Autodesk Inventor part; units mm, degrees
ref_plane "YZ Plane" through (0, 0, 0) normal (1, 0, 0) x (0, 1, 0)
ref_plane "XZ Plane" through (0, 0, 0) normal (0, 1, 0) x (-1, 0, 0)
ref_plane "XY Plane" through (0, 0, 0) normal (0, 0, 1) x (1, 0, 0)
sketch "Sketch1" plane through (0, 0, 0) normal (0, 0, 1) x (1, 0, 0)
  line L0 (0, 0) -> (70, 0)
  line L1 (70, 0) -> (70, 134)
  line L2 (70, 134) -> (0, 134)
  line L3 (0, 134) -> (0, 0)
  dimension "d0" = 70
  dimension "d1" = 134
extrude "Extrusion1" add sketch "Sketch1" along normal blind 3
sketch "Sketch2" plane through (0, 0, 3) normal (0, 0, 1) x (1, 0, 0)
  line L0 (70, 134) -> (0, 134)
  line L1 (0, 134) -> (24, 134)
  line L2 (24, 134) -> (24, 119)
  line L3 (24, 119) -> (0, 119)
  line L4 (0, 119) -> (0, 134)
  line L5 (0, 0) -> (24, 0)
  line L6 (24, 0) -> (24, 15)
  line L7 (24, 15) -> (0, 15)
  line L8 (0, 15) -> (0, 0)
  dimension "d4" = 24
  dimension "d5" = 15
  dimension "d6" = 24
  dimension "d7" = 15
extrude "Extrusion2" add sketch "Sketch2" along normal blind 37
sketch "Sketch3" plane through (0, 0, 40) normal (0, 0, 1) x (1, 0, 0)
  line L0 (24, 134) -> (0, 134) construction
  line L1 (0, 134) -> (0, 119) construction
  line L2 (0, 119) -> (24, 119) construction
  line L3 (24, 119) -> (24, 134) construction
  line L4 (0, 0) -> (24, 0) construction
  line L5 (24, 0) -> (24, 15) construction
  line L6 (24, 15) -> (0, 15) construction
  line L7 (0, 15) -> (0, 0) construction
  circle A0 centre (12, 126.5) radius 1.5
  circle A1 centre (12, 7.5) radius 1.5
  point P0 (24, 126.5)
  point P1 (24, 7.5)
  point P2 (12, 15)
  point P3 (12, 119)
  dimension "d10" = 3
  dimension "d11" = 3
extrude "Extrusion3" cut sketch "Sketch3" against normal through all
sketch "Sketch4" plane through (0, 0, 0) normal (0, 0, -1) x (-1, 0, 0)
  circle A0 centre (-12, 126.5) radius 1.5
  circle A1 centre (-12, 7.5) radius 1.5
  circle A2 centre (-12, 126.5) radius 4
  circle A3 centre (-12, 7.5) radius 4
  point P0 (0, 0)
  dimension "d14" = 8
  dimension "d15" = 8
extrude "Extrusion4" cut sketch "Sketch4" against normal blind 35 contours A0 | A1 | A2 | A3
properties part number "BP009" material "ABS Plastic"
Input: part model. Units: mm. Frame: model coordinates. A direction names the side the tool comes from. Coordinates: 2 decimals unless noted, no trailing zeros. Loops run counter-clockwise (first coordinate to the right, second up) from the corner with the lowest first, then second, coordinate; pieces in that order, holes last.
Q1. Cut plane C-C (x = 12). Output: boundary loops of the cut face in (y, z).
Q2. Set-up query: faces 4 (the face through (24, 7, 21)), 5 (the face through (12, 15, 21)), 6 (the face through (12.1, 5.8, 35)). Return all of +Z, -Z, +X, -X, +Y, -Y with unobstructed straight access to the full face (end or side cutting, diameter ignored); none if empty.
Q3. Material intervals for line 1 (Y direction, x = 12, z = 37.35); line 2 (X direction, y = 126.5, z = 36.35); line 3 (X direction, y = 126, z = 9.5), sorted ascending.
Q4. Cut plane A-A (z = 11). Output: boundary loops of the cut face in (x, y).
Q5. Draft query along Y for faces 1 (the face through (19, 0, 15)), 2 (the face through (35, 68, 3)), 3 (the face through (0, 67, 1)). Return one class per face: +Y half, -Y half, draft (parallel to the pull), parting line (faces both ways), or undercut.
Q6. Cut plane D-D (x = 20.5). Output: boundary loops of the cut face in (y, z), then the cut area to 3 significant figures.
Q7. Cut plane B-B (y = 126.5). Output: boundary loops of the cut face in (x, z), then the cut area to 3 significant figures.
Q8. Contact query for flat-ended pins moving along their axis: pin 1 (5 mm diameter, centred on x = 12, y = 7.5, fed in from +Z); pin 2 (7.5 mm diameter, centred on y = 9, z = 19.5, fed in from +X); pin 3 (2.5 mm diameter, centred on x = 13.5, y = 7, fed in from -Z). Output: stop coordinate, or through.
Working result:
1. outline: (0, 0) - (3.5, 0) - (3.5, 35) - (6, 35) - (6, 40) - (0, 40) - close; (9, 35) - (11.5, 35) - (11.5, 0) - (122.5, 0) - (122.5, 35) - (125, 35) - (125, 40) - (119, 40) - (119, 3) - (15, 3) - (15, 40) - (9, 40) - close; (128, 35) - (130.5, 35) - (130.5, 0) - (134, 0) - (134, 40) - (128, 40) - close
2. face 4: +Z, +X, +Y, -Y
2. face 5: +Z, +X, -X
2. face 6: -Z
3. line 1: y = 0 to 6, 9 to 15, 119 to 125, 128 to 134
3. line 2: x = 0 to 10.5, 13.5 to 24
3. line 3: x = 0 to 8.03, 15.97 to 24
4. outline: (0, 0) - (24, 0) - (24, 15) - (0, 15) - close; (0, 119) - (24, 119) - (24, 134) - (0, 134) - close; hole circle Ø8 at (12, 7.5); hole circle Ø8 at (12, 126.5)
5. face 1: -Y half
5. face 2: undercut
5. face 3: draft
6. outline: (0, 0) - (134, 0) - (134, 40) - (119, 40) - (119, 3) - (15, 3) - (15, 40) - (0, 40) - close
6. area: 1,510 mm2
7. outline: (0, 0) - (8, 0) - (8, 35) - (10.5, 35) - (10.5, 40) - (0, 40) - close; (13.5, 35) - (16, 35) - (16, 0) - (70, 0) - (70, 3) - (24, 3) - (24, 40) - (13.5, 40) - close
7. area: 803 mm2
8. pin 1: stops at z = 40
8. pin 2: stops at x = 24
8. pin 3: stops at z = 35
